```python
from build123d import *

# Parameters (mm, degrees)
SKETCH_1_R            = 3
SKETCH_1_R_2          = 2.75
SKETCH_1_R_3          = 1.7
SKETCH_1_R_4          = 2.5
SKETCH_1_W            = 12
SKETCH_1_H            = 16
F_01_CEILING_M5_DEPTH = 4


with BuildPart() as part:
    # Эскиз1 → 01_Ceiling_M5 (new body)
    with BuildSketch(Plane.XY):
        Polygon((-57, -60), (57, -60), (75, -42), (75, 42), (57, 60), (-57, 60), (-75, 42), (-75, -42), align=None)
        with Locations((-60, -45)):
            Circle(SKETCH_1_R, mode=Mode.SUBTRACT)
        with Locations((-60, 45)):
            Circle(SKETCH_1_R, mode=Mode.SUBTRACT)
        with Locations((60, -45)):
            Circle(SKETCH_1_R_2, mode=Mode.SUBTRACT)
        with Locations((60, 45)):
            Circle(SKETCH_1_R_2, mode=Mode.SUBTRACT)
        with Locations((-36, -25)):
            Circle(SKETCH_1_R_3, mode=Mode.SUBTRACT)
        with Locations((-36, 25)):
            Circle(SKETCH_1_R_3, mode=Mode.SUBTRACT)
        with Locations((36, -25)):
            Circle(SKETCH_1_R_3, mode=Mode.SUBTRACT)
        with Locations((36, 25)):
            Circle(SKETCH_1_R_3, mode=Mode.SUBTRACT)
        with Locations((-53, 0)):
            Circle(SKETCH_1_R_4, mode=Mode.SUBTRACT)
        with Locations((51, 0)):
            Rectangle(SKETCH_1_W, SKETCH_1_H, mode=Mode.SUBTRACT)
    extrude(amount=F_01_CEILING_M5_DEPTH)


solid = part.part
```
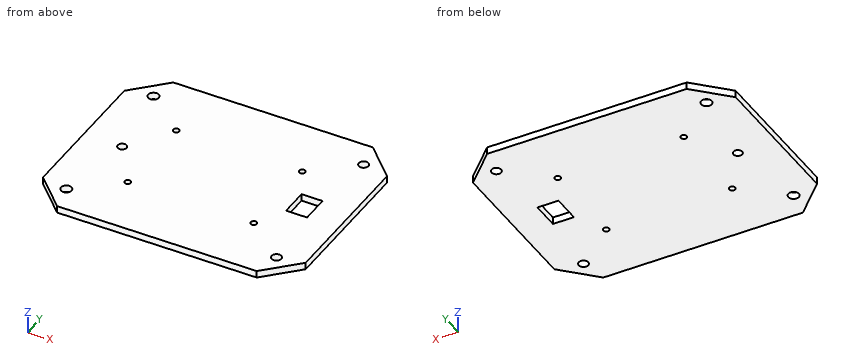
Here's how the part is built. I have some questions about the finished solid (model axes, mm). Give positions to 0.01 mm unless a question says otherwise; leave off trailing zeros. Order: outer loops, then holes, each group sorted by start corner. A loop starts at its lowest first (then second) coordinate and runs counter-clockwise, first axis right, second up. Notation, with made-up numbers: (68, 53) - (85, 53) arc R22 cw to (85, 60) - close; hole circle Ø8 at (82.25, 72.25). An arc over 180 degrees is marked (long way). Answer as a JSON object with one key per item and string values. Group by question number.
Item 1: If we section it at C-C on x = -60: Please give me the cut outline in (y, z), and give its area (3 significant figures).
Item 2: If we section it at B-B on z = 1.5: Give the number of separate pieces and of enclosed holes in the cut face, and give its area (3 significant figures).
Item 3: Please list where these lines run through material, in increasing order: probe 1 along Y at (x, z) = (36, 1.3); probe 2 along Y at (x, z) = (-60, 1.6); probe 3 along X at (y, z) = (44, 1.45).
Item 4: If we section it at A-A on y = 0: Please give me the cut outline in (x, z).
Result set:
{
 "1": {"outline": "(-57, 0) - (-48, 0) - (-48, 4) - (-57, 4) - close; (-42, 0) - (42, 0) - (42, 4) - (-42, 4) - close; (48, 0) - (57, 0) - (57, 4) - (48, 4) - close", "area": "408 mm²"},
 "2": {"separate pieces": "1", "enclosed holes": "10", "area": "17,000 mm²"},
 "3": {"probe 1": "-60 to -26.7, -23.3 to 23.3, 26.7 to 60", "probe 2": "-57 to -48, -42 to 42, 48 to 57", "probe 3": "-73 to -62.83, -57.17 to 57.44, 62.56 to 73"},
 "4": {"outline": "(-75, 0) - (-55.5, 0) - (-55.5, 4) - (-75, 4) - close; (-50.5, 0) - (45, 0) - (45, 4) - (-50.5, 4) - close; (57, 0) - (75, 0) - (75, 4) - (57, 4) - close"}
}
